from build123d import *

# Parameters (mm, degrees)
F0_W     = 101.6
F0_H     = 146.05
F1_DEPTH = 25.4
F2_T     = -2.54
F3_DEPTH = 13.157164678


with BuildPart() as f1:
    # F0 (on Top) → F1 (new body)
    with BuildSketch(Plane.XY):
        with Locations((-8.3804931492, -9.2198206152)):
            Rectangle(F0_W, F0_H)
    extrude(amount=F1_DEPTH)

    # F2
    f2_openings = [f1.faces().sort_by_distance(p)[0] for p in [
        (-8.380493, -9.219821, 25.4),
    ]]
    offset(amount=F2_T, openings=f2_openings)

    # F3 (add): a face of the model
    f3_faces = [f1.faces().sort_by_distance(p)[0] for p in [
        (40.6403732836, -9.2198206152, 25.4),
    ]]
    extrude(f3_faces, amount=F3_DEPTH)


solid = f1.part
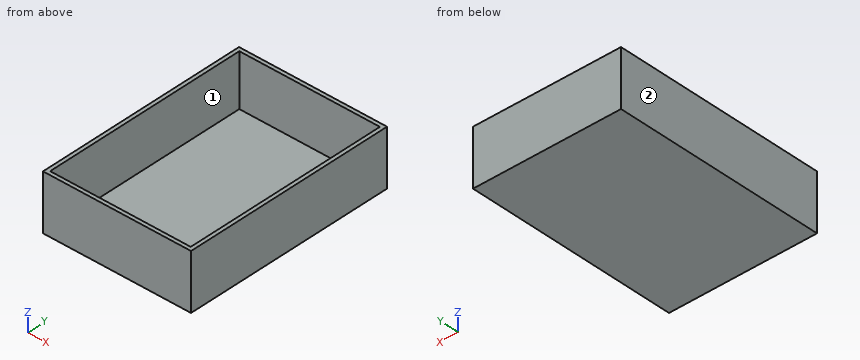
The listing builds one solid part. Answer for the finished solid, in the listing's coordinates (mm). Face numbers are marked on the shaded views. A direction names the side the tool comes from. Give positions to 0.01 mm unless a question says otherwise; leave off trailing zeros. Write each loop counter-clockwise with the first axis right and the second up, starting at its lowest first coordinate (ties: lowest second). Pieces come first, ordered by that corner, then holes.
1) Section A-A (z = 19.5) is taken. Write down the section's boundary in (x, y), and give its area (3 significant figures).
2) Section B-B (x = 17) is taken. Write down the section's boundary in (y, z), and give its area (3 significant figures).
3) Section C-C (y = -50) is taken. Write down the section's boundary in (x, z).
4) Find the intervals of material crossed by L1, parallel to X at y = 1, z = 22; L2, parallel to Y at x = 14, z = 7; L3, parallel to Z at x = -53.5, y = 24, in increasing order.
5) A tool of negligible diameter and unlimited length cuts with its end or side. For the marked faces 1 and 2, from which of +Z, -Z, +X, -X, +Y, -Y can it reach the whole face along a straight path? Write none if from no direction.
6) Given P1, Ø3, axis at x = -16.5, y = 48, coming from the +Z side; P2, Ø8, axis at x = -49, y = -57.5, coming from the -Z side, each flat-ended and moving along its own axis, determine where each tip first touches the part or whether it passes through.
Response:
1. outline: (-59.18, -82.24) - (42.42, -82.24) - (42.42, 63.81) - (-59.18, 63.81) - close; hole (-56.64, -79.7) - (39.88, -79.7) - (39.88, 61.27) - (-56.64, 61.27) - close
1. area: 1,230 mm2
2. outline: (-82.24, 0) - (63.81, 0) - (63.81, 38.56) - (61.27, 38.56) - (61.27, 2.54) - (-79.7, 2.54) - (-79.7, 38.56) - (-82.24, 38.56) - close
2. area: 554 mm2
3. outline: (-59.18, 0) - (42.42, 0) - (42.42, 38.56) - (39.88, 38.56) - (39.88, 2.54) - (-56.64, 2.54) - (-56.64, 38.56) - (-59.18, 38.56) - close
4. L1: x = -59.18 to -56.64, 39.88 to 42.42
4. L2: y = -82.24 to -79.7, 61.27 to 63.81
4. L3: z = 0 to 2.54
5. face 1: +Z
5. face 2: +Z, -Z, -X, +Y, -Y
6. P1: stops at z = 2.54
6. P2: stops at z = 0
